Read the model definition and answer for the solid it produces. Units are mm, in the model's axes. A direction names the side the tool comes from. Give positions to 0.01 mm unless a question says otherwise; leave off trailing zeros. Write each loop counter-clockwise with the first axis right and the second up, starting at its lowest first coordinate (ties: lowest second). Pieces come first, ordered by that corner, then holes. Notation, with made-up numbers: M -8.75,88 L 15.25,88 A15 ccw 15.25,109 Z; hole C 30,52 d6. An arc over 180 degrees is marked long. Use a Markdown table: item, result. Add a question column.
Item 1: A cutting plane is placed at C-C on x = 11.5. Determine the outline of the cut face in (y, z) (3 decimals).
Item 2: A cutting plane is placed at A-A on x = 17.78. Determine the outline of the cut face in (y, z) (3 decimals).
Item 3: Consider probe 1 along Z at (x, y) = (17.78, 2.15); probe 2 along Z at (x, y) = (32, 0.35). Determine where each line is inside the solid, lowest interval first. Write a range as [from, to].
Item 4: A cutting plane is placed at B-B on y = 0.8. Determine the outline of the cut face in (x, z) (3 decimals).
Item 5: The mould has two halves that part along Z. Classify faces 1 (the cylindrical face through (18.051, 1.61, 20.878)), 2 (the flat face through (14.605, 2, 49)), 3 (the flat face through (18, 2, 0)): pulls with the +Z half, pulls with the -Z half, needs draft (parallel to the pull), parting line crosses it, or undercut.
Item 6: Given P1, Ø1.4, axis at y = 1, z = 49, coming from the -X side (3 decimals); P2, Ø1, axis at x = 4.5, y = 1, coming from the +Z side, each flat-ended and moving along its own axis, determine where each tip first touches the part or whether it passes through.
Item 7: For faces 4 (the flat face through (7, 2, 48.006)), 5 (the flat face through (28, 2, 48.006)), 6 (the flat face through (18, 2, 50.8)), determine the directions among +Z, -Z, +X, -X, +Y, -Y from which every point of the face is accessible in a straight line to the end or side of a thin tool.
from build123d import *

# Parameters (mm, degrees)
SKETCH1_W           = 35.56
SKETCH1_H           = 3.175
BOSS_EXTRUDE1_DEPTH = 50.8
SKETCH2_R           = 1.25
CUT_EXTRUDE1_DEPTH  = 63.090532491
SKETCH3_W           = 14.605
SKETCH3_H           = 2.794
CUT_EXTRUDE2_DEPTH  = 63.090532491


with BuildPart() as part:
    # Sketch1 → Boss-Extrude1 (new body)
    with BuildSketch(Plane.XY):
        with Locations((17.78, 1.5875)):
            Rectangle(SKETCH1_W, SKETCH1_H)
    extrude(amount=BOSS_EXTRUDE1_DEPTH)

    # Sketch2 → Cut-Extrude1 (cut, through all)
    with BuildSketch(Plane(origin=(0, 3.175, 0), x_dir=(1, 0, 0), z_dir=(0, 1, 0))):
        with Locations(Location((17.78, -22.098, 0), (0, 0, 180))):
            Circle(SKETCH2_R)
    extrude(amount=-CUT_EXTRUDE1_DEPTH, mode=Mode.SUBTRACT)

    # Sketch3 → Cut-Extrude2 (cut, through all)
    with BuildSketch(Plane(origin=(0, 3.175, 0), x_dir=(1, 0, 0), z_dir=(0, 1, 0))):
        with Locations((7.3025, -49.403)):
            Rectangle(SKETCH3_W, SKETCH3_H)
        with Locations((28.2575, -49.403)):
            Rectangle(SKETCH3_W, SKETCH3_H)
    extrude(amount=-CUT_EXTRUDE2_DEPTH, mode=Mode.SUBTRACT)


solid = part.part
Filled in:
| question | item | result |
|---|---|---|
| 1 | outline | M 0,0 L 3.175,0 L 3.175,48.006 L 0,48.006 Z |
| 2 | outline | M 0,0 L 3.175,0 L 3.175,20.848 L 0,20.848 Z; M 0,23.348 L 3.175,23.348 L 3.175,50.8 L 0,50.8 Z |
| 3 | probe 1 | [0, 20.85], [23.35, 50.8] |
| 3 | probe 2 | [0, 48.01] |
| 4 | outline | M 0,0 L 35.56,0 L 35.56,48.006 L 20.955,48.006 L 20.955,50.8 L 14.605,50.8 L 14.605,48.006 L 0,48.006 Z; hole C 17.78,22.098 d2.5 |
| 5 | face 1 | undercut |
| 5 | face 2 | needs draft |
| 5 | face 3 | pulls with the -Z half |
| 6 | P1 | x = 14.605 |
| 6 | P2 | z = 48.01 |
| 7 | face 4 | +Z, -X, +Y, -Y |
| 7 | face 5 | +Z, +X, +Y, -Y |
| 7 | face 6 | +Z, +X, -X, +Y, -Y |
